```python
from build123d import *

# Parameters (mm, degrees)
PAD_DEPTH         = 10
PAD001_DEPTH      = 5
SKETCH002_W       = 60.350427
SKETCH002_H       = 42.441708
POCKET_DEPTH      = 15.501
POCKET_DEPTH_BACK = -15.501
PAD002_DEPTH      = 7.5
SKETCH004_R       = 7.396265
POCKET001_DEPTH   = 5
SKETCH005_R       = 4.287868
POCKET002_DEPTH   = 18.001
SKETCH006_R       = 7.396265
POCKET003_DEPTH   = 5
POCKET004_DEPTH   = 2
SKETCH008_R       = 5.244286
POCKET005_DEPTH   = 18


with BuildPart() as part:
    # Sketch → Pad (new body)
    with BuildSketch(Plane.XY):
        with BuildLine():
            ThreePointArc((-7.304893, 15.5), (-13.099709, 13.099709), (-15.5, 7.304893))
            Line((-15.5, -7.304893), (-15.5, 7.304893))
            ThreePointArc((-15.5, -7.304893), (-13.099709, -13.099709), (-7.304893, -15.5))
            Line((7.304893, -15.5), (-7.304893, -15.5))
            ThreePointArc((7.304893, -15.5), (13.099709, -13.099709), (15.5, -7.304893))
            Line((15.5, 7.304893), (15.5, -7.304893))
            ThreePointArc((15.5, 7.304893), (13.099709, 13.099709), (7.304893, 15.5))
            Line((-7.304893, 15.5), (7.304893, 15.5))
        make_face()
    extrude(amount=PAD_DEPTH)

    # Sketch001 (on Face4 of Pad) → Pad001 (join, symmetric)
    with BuildSketch(Plane.XZ):
        with BuildLine():
            ThreePointArc((15.5, 17.675132), (0, 33.175132), (-15.5, 17.675132))
            Line((-15.5, 17.675132), (-15.5, -25.955341))
            ThreePointArc((-15.5, -25.955341), (0, -41.455341), (15.5, -25.955341))
            Line((15.5, -25.955341), (15.5, 17.675132))
        make_face()
    extrude(amount=PAD001_DEPTH, both=True)

    # Sketch002 → Pocket (cut, two sides)
    with BuildSketch(Plane.XZ) as pocket_sk:
        with Locations((0.02109, -21.220854)):
            Rectangle(SKETCH002_W, SKETCH002_H)
    extrude(amount=-POCKET_DEPTH, mode=Mode.SUBTRACT)
    extrude(pocket_sk.sketch, amount=-POCKET_DEPTH_BACK, mode=Mode.SUBTRACT)

    # Sketch003 (on Face7 of Pocket) → Pad002 (join, symmetric)
    with BuildSketch(Plane(origin=(0, 0, 0), x_dir=(0, -1, 0), z_dir=(-1, 0, 0))):
        with BuildLine():
            ThreePointArc((-10.127765, -24.385975), (0, -32.810989), (10.127765, -24.385975))
            Line((10.127765, -24.385975), (15.5, 0))
            Line((15.5, 0), (-15.5, 0))
            Line((-10.127765, -24.385975), (-15.5, 0))
        make_face()
    extrude(amount=PAD002_DEPTH, both=True)

    # Sketch004 (on Face10 of Pad002) → Pocket001 (cut)
    with BuildSketch(Plane(origin=(-7.5, 0, 0), x_dir=(0, -1, 0), z_dir=(-1, 0, 0))):
        with Locations((0, -21.767319)):
            Circle(SKETCH004_R)
    extrude(amount=-POCKET001_DEPTH, mode=Mode.SUBTRACT)

    # Sketch005 (on Face34 of Pocket001) → Pocket002 (cut, through all)
    with BuildSketch(Plane(origin=(-2.5, 0, 0), x_dir=(0, -1, 0), z_dir=(-1, 0, 0))):
        with Locations((0, -22.070341)):
            Circle(SKETCH005_R)
    extrude(amount=-POCKET002_DEPTH, mode=Mode.SUBTRACT)

    # Sketch006 (on Face10 of Pad002) → Pocket003 (cut)
    with BuildSketch(Plane(origin=(7.5, 0, 0), x_dir=(0, -1, 0), z_dir=(-1, 0, 0))):
        with Locations((0, -21.767319)):
            Circle(SKETCH006_R)
    extrude(amount=POCKET003_DEPTH, mode=Mode.SUBTRACT)

    # Sketch007 (on Face31 of Pocket003) → Pocket004 (cut)
    with BuildSketch(Plane.XZ.offset(5)):
        Polygon((-6.795665, 30.335199), (-5.335589, 31.015743), (-6.016133, 32.47582), (-7.476209, 31.795276), align=None)
        Polygon((0.805308, 32.018946), (0.805581, 33.629835), (-0.805308, 33.630107), (-0.805581, 32.019218), align=None)
        Polygon((6.794823, 30.3329), (7.475861, 31.792746), (6.016015, 32.473784), (5.334977, 31.013938), align=None)
    extrude(amount=-POCKET004_DEPTH, mode=Mode.SUBTRACT)

    # Sketch008 (on Face31 of Pocket003) → Pocket005 (cut)
    with BuildSketch(Plane.XZ.offset(5)):
        with Locations((-0.002564, 17.667446)):
            Circle(SKETCH008_R)
    extrude(amount=-POCKET005_DEPTH, mode=Mode.SUBTRACT)


solid = part.part
```
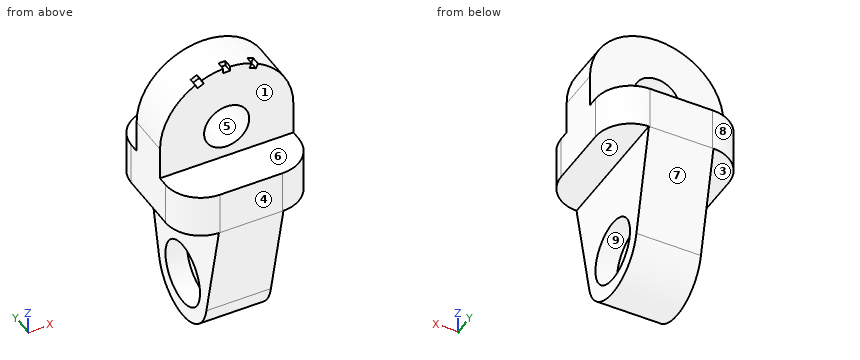
Check sheet for the modelled part. Datum: model origin and axes. Units: mm. Face numbers are marked on the shaded views. A direction names the side the tool comes from. Round coordinates to 2 decimals unless told otherwise and drop trailing zeros. Loops run counter-clockwise (first coordinate to the right, second up) from the corner with the lowest first, then second, coordinate; pieces in that order, holes last. Notation, with made-up numbers: M -17,31.25 L -12,31.25 A17 ccw -12,51.25 Z; hole C 31,55.25 d3. An arc over 180 degrees is marked long. Answer as a JSON object with one key per item and string values.
1. Section check C-C (z = 13.5). Record the boundary of the cut face in (x, y), plus the area to 3 significant figures.
Reply:
{"outline": "M -15.5,-5 L -3.19,-5 L -3.19,5 L -15.5,5 Z; M 3.18,-5 L 15.5,-5 L 15.5,5 L 3.18,5 Z", "area": "246 mm²"}
2. Section check D-D (x = 0). Record the boundary of the cut face in (y, z), plus the area to 3 significant figures.
Reply:
{"outline": "M -15.5,0 L -10.13,-24.39 A10.3 ccw 10.13,-24.39 L 15.5,0 L 15.5,10 L 5,10 L 5,12.42 L -5,12.42 L -5,10 L -15.5,10 Z; M -5,22.91 L 5,22.91 L 5,33.18 L -3,33.18 L -3,32.02 L -5,32.02 Z; hole C 0,-22.07 d8.58", "area": "1,130 mm²"}
3. Section check B-B (x = -4.5). Record the boundary of the cut face in (y, z).
Reply:
{"outline": "M -15.5,0 L -10.13,-24.39 A10.3 ccw 10.13,-24.39 L 15.5,0 L 15.5,10 L 5,10 L 5,14.97 L -5,14.97 L -5,10 L -15.5,10 Z; M -5,20.36 L 5,20.36 L 5,32.51 L -5,32.51 Z; hole C 0,-21.77 d14.79"}
4. Access from +Z, -Z, +X, -X, +Y, -Y to the whole of each face (thin tool, end or side, straight path). Record for the marked faces 1, 2, 3, 4 and 5.
Reply:
{"face 1": "+Z, +X, -X, -Y", "face 2": "-Z, +X, +Y, -Y", "face 3": "-Z, -X, +Y, -Y", "face 4": "+Z, -Z, +X, -X, -Y", "face 5": "+Y, -Y"}
5. Mould release check, pull along Z, two halves, no side actions. Record for the marked faces 6, 7, 8 and 9: pulls with the +Z half, pulls with the -Z half, needs draft (parallel to the pull), parting line crosses it, or undercut.
Reply:
{"face 6": "pulls with the +Z half", "face 7": "pulls with the -Z half", "face 8": "needs draft", "face 9": "undercut"}
6. Gauge pin test, flat ends, axial feed: P1, Ø10, axis at y = 8.5, z = 23.5, coming from the +X side; P2, Ø12, axis at y = 0, z = -21.77, coming from the -X side; P3, Ø3, axis at y = 2, z = -23, coming from the -X side; P4, Ø8, axis at x = 4.5, z = 20, coming from the -Y side. Record the tip position at first contact, or that the pin passes through.
Reply:
{"P1": "stops at x = 15.34", "P2": "stops at x = -2.5", "P3": "passes through", "P4": "stops at y = -5"}
7. Scan lines: line 1 (Z direction, x = 10, y = -7); line 2 (X direction, y = 5, z = -18.5); line 3 (Y direction, x = -9.5, z = 14.5). Record each from-to range of solid material in increasing order.
Reply:
{"line 1": "z = 0 to 10", "line 2": "x = -2.5 to 2.5", "line 3": "y = -5 to 5"}
8. Section check A-A (y = 0). Record the boundary of the cut face in (x, z).
Reply:
{"outline": "M -15.5,0 L -7.5,0 L -7.5,-14.37 L -2.5,-14.37 L -2.5,-17.78 L 2.5,-17.78 L 2.5,-14.37 L 7.5,-14.37 L 7.5,0 L 15.5,0 L 15.5,17.68 A15.5 ccw -15.5,17.68 Z; M -7.5,-32.81 L 7.5,-32.81 L 7.5,-29.16 L 2.5,-29.16 L 2.5,-26.36 L -2.5,-26.36 L -2.5,-29.16 L -7.5,-29.16 Z; hole C 0,17.67 d10.49"}
